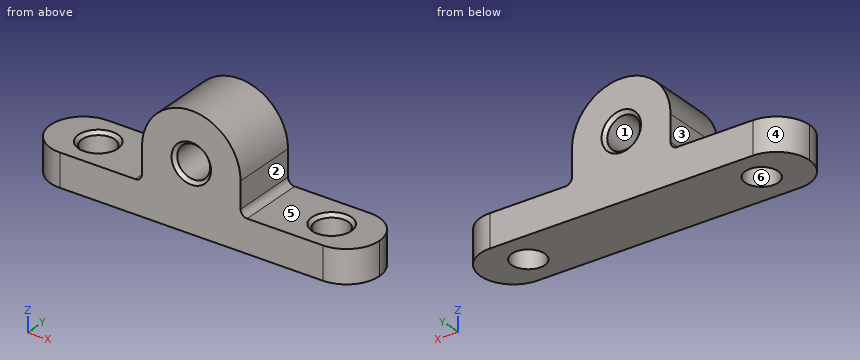
```python
from build123d import *

# Parameters (mm, degrees)
SKETCH1_R               = 1.27
BOSS_EXTRUDE1_DEPTH     = 5.08
FILLET1_R               = 2.54
CUT_EXTRUDE1_DEPTH      = 16.080414451
CUT_EXTRUDE1_DEPTH_BACK = 16.080414451
SKETCH2_R               = 1.27
CHAMFER1_SIZE           = 0.254
FILLET2_R               = 0.508


with BuildPart() as part:
    # Sketch1 → Boss-Extrude1 (new body)
    with BuildSketch(Plane(origin=(0, 0, 0), x_dir=(1, 0, 0), z_dir=(0, 1, 0))):
        with BuildLine():
            Line((-12.7, 5.08), (12.7, 5.08))
            Line((12.7, 5.08), (12.7, 2.54))
            Line((12.7, 2.54), (3.81, 2.54))
            Line((3.81, 2.54), (3.81, 0))
            ThreePointArc((3.81, 0), (0, -3.81), (-3.81, 0))
            Line((-3.81, 0), (-3.81, 2.54))
            Line((-3.81, 2.54), (-12.7, 2.54))
            Line((-12.7, 2.54), (-12.7, 5.08))
        make_face()
        with Locations(Location((0, 0, 0), (0, 0, 270))):
            Circle(SKETCH1_R, mode=Mode.SUBTRACT)
    extrude(amount=BOSS_EXTRUDE1_DEPTH)

    # Fillet1
    fillet1_edges = [part.edges().sort_by_distance(p)[0] for p in [
        (-12.7, 5.08, -3.81),
        (-12.7, 0, -3.81),
        (12.7, 5.08, -3.81),
        (12.7, 0, -3.81),
    ]]
    fillet(fillet1_edges, radius=FILLET1_R - 0.0001)  # a hair under: the kernel refuses the full size

    # Sketch2 → Cut-Extrude1 (cut, two sides: drawn at the far end of the back side and taken through both)
    with BuildSketch(Plane.XY.offset(-2.54).offset(-CUT_EXTRUDE1_DEPTH_BACK)):
        with Locations((-9.017, 2.54)):
            Circle(SKETCH2_R)
        with Locations((9.017, 2.54)):
            Circle(SKETCH2_R)
    extrude(amount=CUT_EXTRUDE1_DEPTH + CUT_EXTRUDE1_DEPTH_BACK, mode=Mode.SUBTRACT)

    # Chamfer1
    chamfer1_edges = [part.edges().sort_by_distance(p)[0] for p in [
        (0, 0, -1.27),
        (0, 5.08, -1.27),
        (-10.287, 2.54, -2.54),
        (7.747, 2.54, -2.54),
    ]]
    chamfer(chamfer1_edges, length=CHAMFER1_SIZE)

    # Fillet2
    fillet2_edges = [part.edges().sort_by_distance(p)[0] for p in [
        (3.81, 2.54, -2.54),
        (-3.81, 2.54, -2.54),
    ]]
    fillet(fillet2_edges, radius=FILLET2_R)


solid = part.part
```
The listing builds one solid part. Answer for the finished solid, in the listing's coordinates (mm). Face numbers are marked on the shaded views. A direction names the side the tool comes from. Coordinates: 2 decimals unless noted, no trailing zeros. Write each loop counter-clockwise with the first axis right and the second up, starting at its lowest first coordinate (ties: lowest second). Pieces come first, ordered by that corner, then holes. Notation, with made-up numbers: (-11, -24.5) - (38, -24.5) arc R28 cw to (38, 9.5) - close; hole circle Ø8 at (34.25, -32.75). An arc over 180 degrees is marked (long way). Return JSON: item names as keys, results as strings. Group by question number.
Q1. For a pull along Y with two mould halves and no side action, classify the marked faces 4, 5 and 6 as +Y half, -Y half, draft (parallel to the pull), parting line (faces both ways), or undercut.
Q2. The part is cut by section B-B on z = -4.5. State how many separate pieces and enclosed holes the cut face has, and give its area (3 significant figures).
Q3. Flat-ended cylindrical pins translate along their axes: pin 1 Ø3 at (x, y) = (-5.5, 3) entering from +Z; pin 2 Ø1.5 at (x, y) = (-9.017, 2.54) entering from -Z; pin 3 Ø1 at (y, z) = (2.5, -1.5) entering from +X; pin 4 Ø1 at (y, z) = (3.5, -3) entering from -X. Find the tip coordinate at first contact, or state that the pin passes through.
Q4. Which of the six approach directions +Z, -Z, +X, -X, +Y, -Y give full straight-line access (tool end or side, diameter ignored) to the marked faces 1, 2 and 3?
Q5. Find the intervals of material crossed by line 1 along X through (y, z) = (2.54, -3.8); line 2 along Z through (x, y) = (-10, 1.05); line 3 along Y through (x, z) = (-8.75, -3.5), in increasing order. Write a range as [from, to].
Q6. The part is cut by section A-A on x = 0. Write down the section's boundary in (y, z).
Q7. The part is cut by section C-C on x = -6.5. Write down the section's boundary in (y, z).
Q8. The part is cut by section D-D on z = 3. Write down the section's boundary in (x, y).
Evaluation:
{
 "1": {"face 4": "+Y half", "face 5": "draft", "face 6": "undercut"},
 "2": {"separate pieces": "1", "enclosed holes": "2", "area": "113 mm2"},
 "3": {"pin 1": "stops at z = -2.43", "pin 2": "passes through", "pin 3": "stops at x = 3.81", "pin 4": "stops at x = -12.66"},
 "4": {"face 1": "+Y, -Y", "face 2": "+Z, +X, +Y, -Y", "face 3": "+Z, -X, +Y, -Y"},
 "5": {"line 1": "x = [-12.7, -10.29], [-7.75, 7.75], [10.29, 12.7]", "line 2": "z = [-5.08, -2.54]", "line 3": "y = [0, 1.3], [3.78, 5.08]"},
 "6": {"outline": "(0, -5.08) - (5.08, -5.08) - (5.08, -1.52) - (4.83, -1.27) - (0.25, -1.27) - (0, -1.52) - close; (0, 1.52) - (0.25, 1.27) - (4.83, 1.27) - (5.08, 1.52) - (5.08, 3.81) - (0, 3.81) - close"},
 "7": {"outline": "(0, -5.08) - (5.08, -5.08) - (5.08, -2.54) - (0, -2.54) - close"},
 "8": {"outline": "(-2.35, 0) - (2.35, 0) - (2.35, 5.08) - (-2.35, 5.08) - close"}
}
